```python
from build123d import *

# Parameters (mm, degrees)
BOSS_EXTRUDE1_DEPTH = 12.7
FILLET1_R           = 2.54
BOSS_EXTRUDE2_DEPTH = 15
SKETCH3_W           = 20.43801088
SKETCH3_H           = 11.408302333
CUT_EXTRUDE1_DEPTH  = 17
FILLET2_R           = 1.27


with BuildPart() as part:
    # Sketch1 → Boss-Extrude1 (new body)
    with BuildSketch(Plane.XY):
        Polygon((0, 0), (0, -4.191), (-1.55575, -4.191), (-1.55575, -7.112), (0, -7.112), (0, -10.287), (10.6045, -10.287), (10.6045, -7.112), (12.16025, -7.112), (12.16025, -4.191), (10.6045, -4.191), (10.6045, 0), (18.97725, 0), (18.97725, 19.558), (15.80225, 19.558), (15.80225, 3.089), (-6.858, 3.089), (-6.858, 0), align=None)
    extrude(amount=BOSS_EXTRUDE1_DEPTH)

    # Fillet1
    fillet1_edges = [part.edges().sort_by_distance(p)[0] for p in [
        (15.80225, 3.089, 6.35),
    ]]
    fillet(fillet1_edges, radius=FILLET1_R)

    # Sketch2 → Boss-Extrude2 (add)
    with BuildSketch(Plane.XY.offset(12.7)):
        Polygon((0, 0), (0, 1.27), (10.6045, 1.27), (10.6045, 0), (10.6045, -4.191), (12.16025, -4.191), (12.16025, -7.112), (10.6045, -7.112), (10.6045, -10.287), (0, -10.287), (0, -7.112), (-1.55575, -7.112), (-1.55575, -4.191), (0, -4.191), align=None)
    extrude(amount=BOSS_EXTRUDE2_DEPTH)

    # Sketch3 → Cut-Extrude1 (cut)
    with BuildSketch(Plane(origin=(0, 0, 0), x_dir=(-1, 0, 0), z_dir=(0, 0, -1))):
        with Locations((-3.189611216, -7.915151167)):
            Rectangle(SKETCH3_W, SKETCH3_H)
    extrude(amount=-CUT_EXTRUDE1_DEPTH, mode=Mode.SUBTRACT)

    # Fillet2
    fillet2_edges = [part.edges().sort_by_distance(p)[0] for p in [
        (5.30225, -2.211, 17),
        (5.30225, 1.27, 12.7),
    ]]
    fillet(fillet2_edges, radius=FILLET2_R)


solid = part.part
```
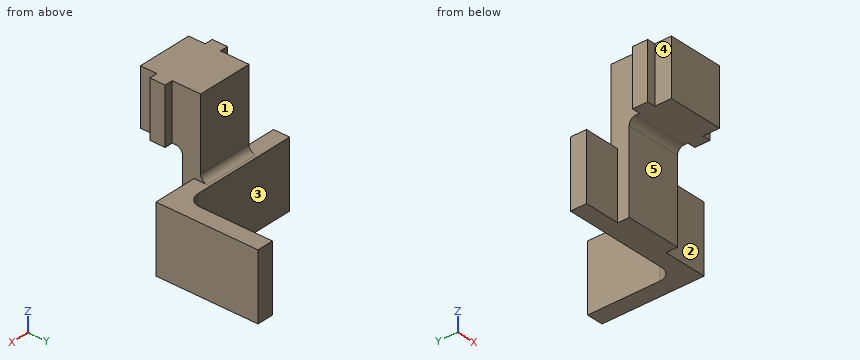
Could you check a few things on this model? Use its own coordinates, in mm. Face numbers are marked on the shaded views. A direction names the side the tool comes from. Coordinates: 2 decimals unless noted, no trailing zeros. Loops run counter-clockwise (first coordinate to the right, second up) from the corner with the lowest first, then second, coordinate; pieces in that order, holes last.
1) Imagine slicing it at B-B (z = 25.5). List the corners of the cut face in (x, y) for me.
Reported:
outline: (-1.56, -7.11) - (0, -7.11) - (0, -10.29) - (10.6, -10.29) - (10.6, -7.11) - (12.16, -7.11) - (12.16, -4.19) - (10.6, -4.19) - (10.6, 1.27) - (0, 1.27) - (0, -4.19) - (-1.56, -4.19) - close
2) Imagine slicing it at A-A (x = -1). List the corners of the cut face in (y, z) for me.
Reported:
outline: (-7.11, 17) - (-4.19, 17) - (-4.19, 27.7) - (-7.11, 27.7) - close; (0, 0) - (3.09, 0) - (3.09, 12.7) - (0, 12.7) - close
3) Will these pins go through, and if not, where does the flat tip stop? pin 1 Ø4 at (x, z) = (-1.5, 6.5) entering from -Y; pin 2 Ø1.5 at (y, z) = (-6.5, 20) entering from +X; pin 3 Ø0.5 at (x, z) = (-1, 20) entering from +Y.
Reported:
pin 1: stops at y = -2.21
pin 2: stops at x = 12.16
pin 3: stops at y = -4.19
4) Imagine slicing it at C-C (y = -7.75). List the corners of the cut face in (x, z) for me.
Reported:
outline: (0, 17) - (10.6, 17) - (10.6, 27.7) - (0, 27.7) - close
5) Which directions (+Z, -Z, +X, -X, +Y, -Y) give clear straight access to the entire face, cutting with the end or side of a thin tool? Please do the marked faces 1, 2, 3, 4 and 5.
Reported:
face 1: +Z, +X, -X, +Y
face 2: +Z, -Z, +X, -Y
face 3: +Z, -Z, -X, +Y
face 4: +Z, -Z, -X, -Y
face 5: -Z, +X, -X, -Y
6) Please list where these lines run through material, in increasing order: line 1 along Y through (x, z) = (-6, 7.5); line 2 along Z through (x, y) = (-1, 1); line 3 along Y through (x, z) = (2, 20.75).
Reported:
line 1: y = 0 to 3.09
line 2: z = 0 to 12.7
line 3: y = -10.29 to 1.27
7) Imagine slicing it at D-D (x = 4.75). List the corners of the cut face in (y, z) for me.
Reported:
outline: (-10.29, 17) - (-3.48, 17) arc R1.27 cw to (-2.21, 15.73) - (-2.21, 0) - (3.09, 0) - (3.09, 12.7) - (2.54, 12.7) arc R1.27 cw to (1.27, 13.97) - (1.27, 27.7) - (-10.29, 27.7) - close
